The model under review builds one solid part; all positions refer to its coordinate system, in mm. A direction names the side the tool comes from. Coordinates: 2 decimals unless noted, no trailing zeros. Loops run counter-clockwise (first coordinate to the right, second up) from the corner with the lowest first, then second, coordinate; pieces in that order, holes last. Notation, with made-up numbers: M 60.25,-15 L 111.25,-15 A23 ccw 111.25,11 Z; hole C 64,-28.75 d5. An arc over 180 degrees is marked long. Use CSV: the item, a comma, the result in double quotes. Start each with the question number.
1. Add section B-B, the plane x = 2.5. Write out the cut boundary in (y, z), then the cut area to 3 significant figures.
2. For L1, parallel to Y at x = 2.75, z = 0.25; L2, parallel to X at y = 6.5, z = 1; L3, parallel to X at y = 28, z = -1, list the stretches that pass through material, from the lowest coordinate up.
3. Add section C-C, the plane y = 7. Write out the cut boundary in (x, z), then the cut area to 3 significant figures.
4. Add section A-A, the plane y = 25.5. Write out the cut boundary in (x, z) (3 decimals).
5. Clearance check with a flat-ended pin moving along its axis: P1, Ø3, axis at y = 20.5, z = 0.5, coming from the +X side (3 decimals). State where the tip first meets the part, or that it passes through.
6. Tool access review of faces 1 (the flat face through (2.3, 15, 0)), 2 (the cylindrical face through (-0.45, 5.92, -1.43)), 3 (the flat face through (2.6, 13.5, -1.5)): name each direction out of +Z, -Z, +X, -X, +Y, -Y from which nothing blocks a thin tool from reaching the whole face with its end or side.
from build123d import *

# Parameters (mm, degrees)
BOSS_EXTRUDE1_DEPTH = 3
CHAMFER1_SIZE       = 1


with BuildPart() as part:
    # Sketch1 → Revolve1 (revolve)
    with BuildSketch(Plane.XY, mode=Mode.PRIVATE) as revolve1_sk:
        Polygon((0, 34), (-1.905, 34), (-1.905, 15), (-2.5, 15), (-2.5, 12), (-1.5, 12), (-1.5, 0), (0, 0), align=None)
    revolve(revolve1_sk.sketch.rotate(Axis((0, 0, 0), (0, 1, 0)), 270), axis=Axis((0, 0, 0), (0, 1, 0)))

    # Sketch2 → Boss-Extrude1 (add)
    with BuildSketch(Plane(origin=(0, 15, 0), x_dir=(1, 0, 0), z_dir=(0, 1, 0))):
        Polygon((-3.464101615, 0), (-1.732050808, -3), (1.732050808, -3), (3.464101615, 0), (1.732050808, 3), (-1.732050808, 3), align=None)
    extrude(amount=-BOSS_EXTRUDE1_DEPTH)

    # Chamfer1
    chamfer1_edges = [part.edges().sort_by_distance(p)[0] for p in [
        (0, 34, 1.905),
    ]]
    chamfer(chamfer1_edges, length=CHAMFER1_SIZE)


solid = part.part
Computed:
1,outline,"M 12,-1.67 L 15,-1.67 L 15,1.67 L 12,1.67 Z"
1,area,"10.0 mm^2"
2,L1,"y = 12 to 15"
2,L2,"x = -1.12 to 1.12"
2,L3,"x = -1.62 to 1.62"
3,outline,"C 0,0 d3"
3,area,"7.07 mm^2"
4,outline,"C 0,0 d3.81"
5,P1,"stops at x = 1.905"
6,face 1,"+Y"
6,face 2,"-Y"
6,face 3,"-Z, +X, +Y, -Y"
